Build history of the part. All positions in model axes, mm. Give positions to 0.01 mm unless a question says otherwise; leave off trailing zeros. Write each loop counter-clockwise with the first axis right and the second up, starting at its lowest first coordinate (ties: lowest second). Pieces come first, ordered by that corner, then holes.
from build123d import *

# Parameters (mm, degrees)
F0_W         = 508
F0_H         = 12.7
F0_R         = 1.5875
F1_DEPTH     = 6.35
F2_T1_DEPTH  = 540.6603739472
F3_T1_DEPTH  = 8.3226920908
F3_T3_DEPTH  = 8.0055929849
F3_T5_DEPTH  = 5.2274679849
F3_T7_DEPTH  = 13.890625
F3_T9_DEPTH  = 8.3226920908
F3_T11_DEPTH = 506.4125
F3_T13_DEPTH = 11.1407050378
F3_T15_DEPTH = 36.5689100757
F3_T17_DEPTH = 11.1407050378
F3_T22_DEPTH = 0.809625
F3_T28_DEPTH = 0.809625
F3_S33_W     = 0.809625
F3_S33_H     = 0.809625
F3_T34_DEPTH = 0.809625
F3_T40_DEPTH = 0.809625
F3_T46_DEPTH = 0.809625
F3_S51_W     = 0.809625
F3_S51_H     = 0.809625
F3_T52_DEPTH = 0.809625


# Not quite as in the source:
# - a fillet or chamfer that OpenCascade refuses, or shapes differently, is made with other operations: its cross-section is extruded or revolved along the edge and cut away or added


with BuildPart() as f1:
    # F0 (on Top) → F1 (new body, symmetric)
    with BuildSketch(Plane.XY):
        with Locations((4.392349353, 0)):
            Rectangle(F0_W, F0_H)
        with Locations((-236.907650647, 0)):
            Circle(F0_R, mode=Mode.SUBTRACT)
        with Locations((-198.807650647, 0)):
            Circle(F0_R, mode=Mode.SUBTRACT)
        with Locations((207.592349353, 0)):
            Circle(F0_R, mode=Mode.SUBTRACT)
        with Locations((245.692349353, 0)):
            Circle(F0_R, mode=Mode.SUBTRACT)
    extrude(amount=F1_DEPTH, both=True)

    # F2: chamfer of 6.35 on 1 edges, made by hand

    # F2_s2 → F2_t1 (cut)
    with BuildSketch(Plane.YZ.offset(-265.9378376206)):
        Polygon((-6.35, 0), (0, -6.35), (-6.35, -6.35), align=None)
    extrude(amount=F2_T1_DEPTH, mode=Mode.SUBTRACT)

    # F3: fillet of radius 0.79375 on 13 edges, made by hand

    # F3_s2 → F3_t1 (cut)
    with BuildSketch(Plane(origin=(0, 2.9425160076, -2.9425160076), x_dir=(1, 0, 0), z_dir=(0, -0.7071067812, 0.7071067812))):
        with BuildLine():
            ThreePointArc((258.392349353, -3.6963780605), (258.1598653606, -4.2576440681), (257.598599353, -4.4901280605))
            Line((257.598599353, -4.4901280605), (258.392349353, -4.4901280605))
            Line((258.392349353, -4.4901280605), (258.392349353, -3.6963780605))
        make_face()
    extrude(amount=F3_T1_DEPTH, mode=Mode.SUBTRACT)

    # F3_s4 → F3_t3 (cut)
    with BuildSketch(Plane.XY.offset(0.3287820151)):
        with BuildLine():
            ThreePointArc((258.392349353, -5.55625), (258.1598653606, -6.1175160076), (257.598599353, -6.35))
            Line((257.598599353, -6.35), (258.392349353, -6.35))
            Line((258.392349353, -6.35), (258.392349353, -5.55625))
        make_face()
        with BuildLine():
            ThreePointArc((-249.607650647, -5.55625), (-249.3751666546, -6.1175160076), (-248.813900647, -6.35))
            Line((-248.813900647, -6.35), (-249.607650647, -6.35))
            Line((-249.607650647, -6.35), (-249.607650647, -5.55625))
        make_face()
    extrude(amount=F3_T3_DEPTH, mode=Mode.SUBTRACT)

    # F3_s6 → F3_t5 (cut)
    with BuildSketch(Plane.XZ.offset(-5.55625)):
        with BuildLine():
            ThreePointArc((257.598599353, -6.35), (258.1598653606, -6.1175160076), (258.392349353, -5.55625))
            Line((258.392349353, -5.55625), (258.392349353, -6.35))
            Line((258.392349353, -6.35), (257.598599353, -6.35))
        make_face()
        with BuildLine():
            ThreePointArc((-248.813900647, -6.35), (-249.3751666546, -6.1175160076), (-249.607650647, -5.55625))
            Line((-249.607650647, -5.55625), (-249.607650647, -6.35))
            Line((-249.607650647, -6.35), (-248.813900647, -6.35))
        make_face()
    extrude(amount=F3_T5_DEPTH, mode=Mode.SUBTRACT)

    # F3_s8 → F3_t7 (cut)
    with BuildSketch(Plane.XY.offset(-5.55625)):
        with BuildLine():
            ThreePointArc((257.598599353, 6.35), (258.1598653606, 6.1175160076), (258.392349353, 5.55625))
            Line((258.392349353, 5.55625), (258.392349353, 6.35))
            Line((258.392349353, 6.35), (257.598599353, 6.35))
        make_face()
        with BuildLine():
            ThreePointArc((-248.813900647, 6.35), (-249.3751666546, 6.1175160076), (-249.607650647, 5.55625))
            Line((-249.607650647, 5.55625), (-249.607650647, 6.35))
            Line((-249.607650647, 6.35), (-248.813900647, 6.35))
        make_face()
    extrude(amount=F3_T7_DEPTH, mode=Mode.SUBTRACT)

    # F3_s10 → F3_t9 (cut)
    with BuildSketch(Plane(origin=(0, -2.9425160076, 2.9425160076), x_dir=(1, 0, 0), z_dir=(0, 0.7071067812, -0.7071067812))):
        with BuildLine():
            ThreePointArc((-249.607650647, 3.6963780605), (-249.3751666546, 4.2576440681), (-248.813900647, 4.4901280605))
            Line((-248.813900647, 4.4901280605), (-249.607650647, 4.4901280605))
            Line((-249.607650647, 4.4901280605), (-249.607650647, 3.6963780605))
        make_face()
    extrude(amount=F3_T9_DEPTH, mode=Mode.SUBTRACT)

    # F3_s12 → F3_t11 (cut)
    with BuildSketch(Plane.YZ.offset(-248.813900647)):
        with BuildLine():
            ThreePointArc((-6.1175160076, -0.2324839924), (-6.2895793789, 0.0250270407), (-6.35, 0.3287820151))
            Line((-6.35, 0.3287820151), (-6.35, 0))
            Line((-6.35, 0), (-6.1175160076, -0.2324839924))
        make_face()
        with BuildLine():
            ThreePointArc((6.35, -5.55625), (6.1175160076, -6.1175160076), (5.55625, -6.35))
            Line((5.55625, -6.35), (6.35, -6.35))
            Line((6.35, -6.35), (6.35, -5.55625))
        make_face()
    extrude(amount=F3_T11_DEPTH, mode=Mode.SUBTRACT)

    # F3_s14 → F3_t13 (cut)
    with BuildSketch(Plane.YZ.offset(-248.813900647)):
        with BuildLine():
            ThreePointArc((0.3287820151, -6.35), (0.0250270407, -6.2895793789), (-0.2324839924, -6.1175160076))
            Line((-0.2324839924, -6.1175160076), (0, -6.35))
            Line((0, -6.35), (0.3287820151, -6.35))
        make_face()
    extrude(amount=F3_T13_DEPTH, mode=Mode.SUBTRACT)

    # F3_s16 → F3_t15 (cut)
    with BuildSketch(Plane.YZ.offset(-236.1421056848)):
        with BuildLine():
            ThreePointArc((0.3287820151, -6.35), (0.0250270407, -6.2895793789), (-0.2324839924, -6.1175160076))
            Line((-0.2324839924, -6.1175160076), (0, -6.35))
            Line((0, -6.35), (0.3287820151, -6.35))
        make_face()
    extrude(amount=F3_T15_DEPTH, mode=Mode.SUBTRACT)

    # F3_s18 → F3_t17 (cut)
    with BuildSketch(Plane.YZ.offset(246.4578943152)):
        with BuildLine():
            ThreePointArc((0.3287820151, -6.35), (0.0250270407, -6.2895793789), (-0.2324839924, -6.1175160076))
            Line((-0.2324839924, -6.1175160076), (0, -6.35))
            Line((0, -6.35), (0.3287820151, -6.35))
        make_face()
    extrude(amount=F3_T17_DEPTH, mode=Mode.SUBTRACT)


with BuildPart() as f3_tool20:
    # F3_s21 → F3_t22 (new body)
    with BuildSketch(Plane.YZ.offset(257.598599353)):
        Polygon((0.3287820151, -5.55625), (-0.2437093126, -6.1287413277), (-0.0065756403, -6.365875), (0.3287820151, -6.365875), align=None)
    extrude(amount=F3_T22_DEPTH)

    # F3_s23 → F3_t24 (revolve, cut)
    with BuildSketch(Plane(origin=(257.598599353, 0.3287820151, -5.55625), x_dir=(0, 0.3826834324, 0.9238795325), z_dir=(0, 0.9238795325, -0.3826834324))):
        with BuildLine():
            ThreePointArc((0, -0.79375), (0.79375, 0), (0, 0.79375))
            Line((0, 0.79375), (0, -0.79375))
        make_face()
    revolve(axis=Axis((257.598599353, 0.3287820151, -5.55625), (1, 0, 0)), mode=Mode.SUBTRACT)


with BuildPart() as f1_1:
    add(f1.part)

    # F3_t19: cut F3_tool20
    add(f3_tool20.part, mode=Mode.SUBTRACT)


with BuildPart() as f3_tool26:
    # F3_s27 → F3_t28 (new body)
    with BuildSketch(Plane.YZ.offset(257.598599353)):
        Polygon((-5.55625, 0.3287820151), (-6.1287413277, -0.2437093126), (-6.365875, -0.0065756403), (-6.365875, 0.3287820151), align=None)
    extrude(amount=F3_T28_DEPTH)

    # F3_s29 → F3_t30 (revolve, cut)
    with BuildSketch(Plane(origin=(257.598599353, -5.55625, 0.3287820151), x_dir=(0, 0.9238795325, 0.3826834324), z_dir=(0, 0.3826834324, -0.9238795325))):
        with BuildLine():
            ThreePointArc((0, -0.79375), (0.79375, 0), (0, 0.79375))
            Line((0, 0.79375), (0, -0.79375))
        make_face()
    revolve(axis=Axis((257.598599353, -5.55625, 0.3287820151), (1, 0, 0)), mode=Mode.SUBTRACT)


with BuildPart() as f1_2:
    add(f1_1.part)

    # F3_t25: cut F3_tool26
    add(f3_tool26.part, mode=Mode.SUBTRACT)


with BuildPart() as f3_tool32:
    # F3_s33 → F3_t34 (new body)
    with BuildSketch(Plane.XZ.offset(-5.55625)):
        with Locations((258.003411853, -5.9610625)):
            Rectangle(F3_S33_W, F3_S33_H)
    extrude(amount=-F3_T34_DEPTH)

    # F3_s35 → F3_t36 (revolve, cut)
    with BuildSketch(Plane(origin=(257.598599353, 5.55625, -5.55625), x_dir=(-0.7071067812, 0, 0.7071067812), z_dir=(-0.7071067812, 0, -0.7071067812))):
        with BuildLine():
            ThreePointArc((0, -0.79375), (0.79375, 0), (0, 0.79375))
            Line((0, 0.79375), (0, -0.79375))
        make_face()
    revolve(axis=Axis((257.598599353, 5.55625, -5.55625), (0, 1, 0)), mode=Mode.SUBTRACT)


with BuildPart() as f1_3:
    add(f1_2.part)

    # F3_t31: cut F3_tool32
    add(f3_tool32.part, mode=Mode.SUBTRACT)


with BuildPart() as f3_tool38:
    # F3_s39 → F3_t40 (new body)
    with BuildSketch(Plane.YZ.offset(-248.813900647)):
        Polygon((-5.55625, 0.3287820151), (-6.365875, 0.3287820151), (-6.365875, -0.0065756403), (-6.1287413277, -0.2437093126), align=None)
    extrude(amount=-F3_T40_DEPTH)

    # F3_s41 → F3_t42 (revolve, cut)
    with BuildSketch(Plane(origin=(-248.813900647, -5.55625, 0.3287820151), x_dir=(0, 0.9238795325, 0.3826834324), z_dir=(0, -0.3826834324, 0.9238795325))):
        with BuildLine():
            ThreePointArc((0, -0.79375), (0.79375, 0), (0, 0.79375))
            Line((0, 0.79375), (0, -0.79375))
        make_face()
    revolve(axis=Axis((-248.813900647, -5.55625, 0.3287820151), (-1, 0, 0)), mode=Mode.SUBTRACT)


with BuildPart() as f1_4:
    add(f1_3.part)

    # F3_t37: cut F3_tool38
    add(f3_tool38.part, mode=Mode.SUBTRACT)


with BuildPart() as f3_tool44:
    # F3_s45 → F3_t46 (new body)
    with BuildSketch(Plane.YZ.offset(-248.813900647)):
        Polygon((0.3287820151, -5.55625), (-0.2437093126, -6.1287413277), (-0.0065756403, -6.365875), (0.3287820151, -6.365875), align=None)
    extrude(amount=-F3_T46_DEPTH)

    # F3_s47 → F3_t48 (revolve, cut)
    with BuildSketch(Plane(origin=(-248.813900647, 0.3287820151, -5.55625), x_dir=(0, 0.3826834324, 0.9238795325), z_dir=(0, -0.9238795325, 0.3826834324))):
        with BuildLine():
            ThreePointArc((0, -0.79375), (0.79375, 0), (0, 0.79375))
            Line((0, 0.79375), (0, -0.79375))
        make_face()
    revolve(axis=Axis((-248.813900647, 0.3287820151, -5.55625), (-1, 0, 0)), mode=Mode.SUBTRACT)


with BuildPart() as f1_5:
    add(f1_4.part)

    # F3_t43: cut F3_tool44
    add(f3_tool44.part, mode=Mode.SUBTRACT)


with BuildPart() as f3_tool50:
    # F3_s51 → F3_t52 (new body)
    with BuildSketch(Plane.XZ.offset(-5.55625)):
        with Locations((-249.218713147, -5.9610625)):
            Rectangle(F3_S51_W, F3_S51_H)
    extrude(amount=-F3_T52_DEPTH)

    # F3_s53 → F3_t54 (revolve, cut)
    with BuildSketch(Plane(origin=(-248.813900647, 5.55625, -5.55625), x_dir=(0.7071067812, 0, 0.7071067812), z_dir=(-0.7071067812, 0, 0.7071067812))):
        with BuildLine():
            ThreePointArc((0, -0.79375), (0.79375, 0), (0, 0.79375))
            Line((0, 0.79375), (0, -0.79375))
        make_face()
    revolve(axis=Axis((-248.813900647, 5.55625, -5.55625), (0, 1, 0)), mode=Mode.SUBTRACT)


with BuildPart() as f1_6:
    add(f1_5.part)

    # F3_t49: cut F3_tool50
    add(f3_tool50.part, mode=Mode.SUBTRACT)


solid = f1_6.part
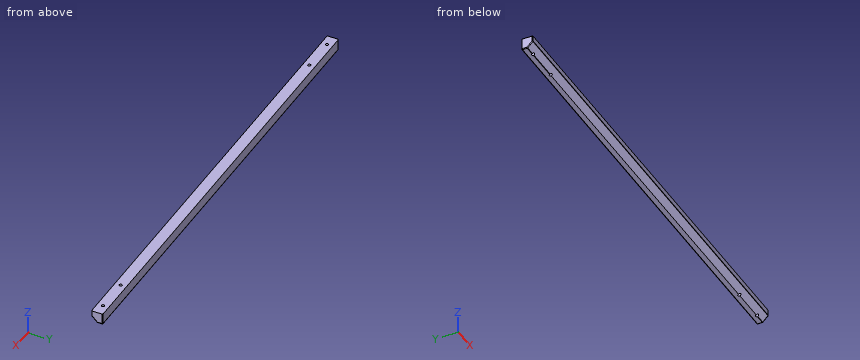
(1) Saw through at A-A, the plane x = -80. List the corners of the cut face in (y, z).
(2) Drop flat-ended pins along their axis: pin 1 (4 mm diameter, centred on x = -236.91, y = 0, fed in from -Z); pin 2 (2.5 mm diameter, centred on x = 207.59, y = 0, fed in from -Z); pin 3 (1.5 mm diameter, centred on y = -3, z = -4, fed in from +X). Give the stop position or say it passes through.
(3) Probe line 1 (X direction, y = -0.5, z = -2.25); line 2 (X direction, y = 0, z = 0.75); line 3 (Z direction, x = -147, y = -2). List the from-to ranges inside material, lowest first.
Computed values:
1. outline: (-6.35, 0.33) arc R0.79 ccw to (-6.12, -0.23) - (0, -6.35) - (5.56, -6.35) arc R0.79 ccw to (6.35, -5.56) - (6.35, 6.35) - (-6.35, 6.35) - close
2. pin 1: stops at z = -6.35
2. pin 2: passes through
2. pin 3: stops at x = 258.21
3. line 1: x = -249.61 to -238.41, -235.4 to -200.31, -197.3 to 206.09, 209.1 to 244.19, 247.2 to 258.39
3. line 2: x = -249.61 to -238.5, -235.32 to -200.4, -197.22 to 206, 209.18 to 244.1, 247.28 to 258.39
3. line 3: z = -4.35 to 6.35
